Input: part model. Units: mm. Frame: model coordinates. A direction names the side the tool comes from. Coordinates: 2 decimals unless noted, no trailing zeros. Order: outer loops, then holes, each group sorted by start corner. A loop starts at its lowest first (then second) coordinate and runs counter-clockwise, first axis right, second up. Notation, with made-up numbers: M -28.75,17.25 L 22.25,17.25 A21 ccw 22.25,24.25 Z; hole C 77,-30.75 d3. An arc over 180 degrees is marked long. One line per item, written item: value.
Autodesk Inventor part; units mm, degrees
ref_plane "YZ Plane" through (0, 0, 0) normal (1, 0, 0) x (0, 1, 0)
ref_plane "XZ Plane" through (0, 0, 0) normal (0, 1, 0) x (-1, 0, 0)
ref_plane "XY Plane" through (0, 0, 0) normal (0, 0, 1) x (1, 0, 0)
sketch "スケッチ1" plane through (0, 0, 0) normal (0, 0, 1) x (1, 0, 0)
  line L0 (0, 0) -> (0, 51.1276) construction
  line L1 (-6, 43) -> (6, 43) construction
  arc A0 (9, 40) -> (6, 43) centre (6, 40) ccw
  line L2 (9, 40) -> (9, 36.5)
  line L3 (10.5, 35) -> (12.5, 35)
  arc A1 (14, 33.5) -> (12.5, 35) centre (12.5, 33.5) ccw
  line L4 (14, 0) -> (14, 33.5) construction
  line L5 (10, 47) -> (-10, 47) construction
  line L6 (16, 40) -> (10, 47) construction
  line L7 (16, 26.6395) -> (16, 40) construction
  circle A2 centre (12.5, 38.5) radius 1.5 construction
  circle A3 centre (17.5, 20) radius 1.5 construction
  line L8 (22.5, 39.5) -> (22.5, 0.5)
  line L9 (22, 0) -> (14.5, 0)
  arc A4 (20.6, 30.9506) -> (17.4, 30.9506) centre (19, 33) ccw
  arc A5 (17.4, 29) -> (20.6, 29) centre (19, 29) ccw
  line L10 (17.4, 30.9506) -> (17.4, 29)
  line L11 (20.6, 30.9506) -> (20.6, 29)
  line L12 (19, 29) -> (19, 33) construction
  line L13 (10, 47) -> (16, 40)
  arc A6 (17.4, 7) -> (20.6, 7) centre (19, 7) ccw
  line L14 (17.4, 7) -> (17.4, 8.9506)
  line L15 (20.6, 7) -> (20.6, 8.9506)
  arc A7 (20.6, 8.9506) -> (17.4, 8.9506) centre (19, 11) ccw
  line L16 (19, 11) -> (19, 7) construction
  line L17 (14, 33.5) -> (14, 0.5)
  line L18 (0, 43) -> (0, 47)
  line L19 (0, 47) -> (10, 47)
  line L20 (6, 43) -> (0, 43)
  line L21 (16, 40) -> (22, 40)
  line L22 (22, 40) -> (22.5, 39.5)
  line L23 (22, 0) -> (22.5, 0.5)
  circle A8 centre (17.5, 20) radius 1.05
  circle A9 centre (12.5, 38.5) radius 1.05
  arc A10 (9, 36.5) -> (10.5, 35) centre (10.5, 36.5) ccw
  line L24 (14, 0.5) -> (14.5, 0)
  point P0 (22.5, 40)
  point P1 (22.5, 0)
  dimension "d5" = 2.6
  dimension "d6" = 4
  dimension "d10" = 4
  dimension "d14" = 0.5
  dimension "d15" = 0.5
  dimension "d17" = 0.5
  dimension "d18" = 0.5
  dimension "d19" = 2.1
  dimension "d20" = 9
  dimension "d21" = 9
  dimension "d22" = 2.1
  dimension "d23" = 1.5
  dimension "d24" = 1.6
  dimension "d25" = 2.6
  dimension "d26" = 1.6
  dimension "d28" = 38
  dimension "d29" = 45
  dimension "d30" = 40
  dimension "d31" = 0.5
  dimension "d32" = 0.5
  dimension "d36" = 28
  dimension "d37" = 10
  dimension "d38" = 6
  dimension "d39" = 7
extrude "押し出し1" add sketch "スケッチ1" along normal blind 2
sketch "スケッチ3" plane through (0, 0, 2) normal (0, 0, 1) x (1, 0, 0)
  circle A0 centre (17.5, 20) radius 1.05
  circle A1 centre (17.5, 20) radius 1.8
  circle A2 centre (12.5, 38.5) radius 1.05
  circle A3 centre (12.5, 38.5) radius 1.8
  point P0 (0, 0)
  dimension "d33" = 3.6
extrude "押し出し2" cut sketch "スケッチ3" against normal blind 0.8
mirror "ミラー1" about plane through (0, 0, 0) normal (1, 0, 0) of "押し出し1", "押し出し2"
properties part number "16_035_BATTERY_HOLDER_BACK_R1"
(1) Cut plane B-B on y = 11. Output: boundary loops of the cut face in (x, z), plus the area to 3 significant figures.
Data:
outline: M -22.5,0 L -21.6,0 L -21.6,2 L -22.5,2 Z; M -16.4,0 L -14,0 L -14,2 L -16.4,2 Z; M 14,0 L 16.4,0 L 16.4,2 L 14,2 Z; M 21.6,0 L 22.5,0 L 22.5,2 L 21.6,2 Z
area: 13.2 mm2
(2) Ray query, line 1 (X direction, y = 11, z = 1.4); line 2 (X direction, y = 25, z = 1.1); line 3 (X direction, y = 31.5, z = 0.7). Return the intervals inside material, ascending. Write a range as from..to.
Data:
line 1: x = -22.5..-21.6, -16.4..-14, 14..16.4, 21.6..22.5
line 2: x = -22.5..-14, 14..22.5
line 3: x = -22.5..-21.12, -16.88..-14, 14..16.88, 21.12..22.5
(3) First-contact query: pin 1 (1 mm diameter, centred on x = 11.5, z = 1, fed in from -Y); pin 2 (3.5 mm diameter, centred on x = 17.5, y = 20, fed in from -Z); pin 3 (1 mm diameter, centred on x = -14.5, z = 1, fed in from +Y); pin 4 (1 mm diameter, centred on x = 19, z = 1, fed in from +Y). Flat tips, straight axial feed; report the tip coordinate or a pass-through.
Data:
pin 1: stops at y = 35
pin 2: stops at z = 0
pin 3: stops at y = 42.33
pin 4: stops at y = 40
(4) Cut plane A-A on y = 4. Output: boundary loops of the cut face in (x, z).
Data:
outline: M -22.5,0 L -14,0 L -14,2 L -22.5,2 Z; M 14,0 L 22.5,0 L 22.5,2 L 14,2 Z
(5) Cut plane C-C on x = -2.5. Output: boundary loops of the cut face in (y, z).
Data:
outline: M 43,0 L 47,0 L 47,2 L 43,2 Z
(6) Cut plane D-D on z = 0.75. Give the number of separate pieces and of enclosed holes in the cut face, plus the area to 3 significant figures.
Data:
separate pieces: 1
enclosed holes: 8
area: 726 mm2
(7) Draft query along X for faces 4 (the flat face through (-17.4, 8, 1)), 5 (the flat face through (0, 47, 1)), 6 (the flat face through (-22.5, 20, 1)), 7 (the cylindrical face through (-11.173, 37.283, 1.606)). Return one class per face: released by +X, released by -X, zero draft, split by the parting line, or undercut.
Data:
face 4: undercut
face 5: zero draft
face 6: released by -X
face 7: undercut
(8) Access query for faces 1 (the cylindrical face through (12.266, 40.285, 1.606)), 2 (the flat face through (-20.6, 8, 1)), 3 (the cylindrical face through (-8.14, 42.1, 0.99)). Directions: +Z, -Z, +X, -X, +Y, -Y. A direction counts if a zero-diameter tool reaches every point of the face in a straight line with its end or side. Return the directions, or none.
Data:
face 1: +Z
face 2: +Z, -Z
face 3: +Z, -Z, -Y
